The model under review builds one solid part; all positions refer to its coordinate system, in mm. A direction names the side the tool comes from. Give positions to 0.01 mm unless a question says otherwise; leave off trailing zeros. Loops run counter-clockwise (first coordinate to the right, second up) from the corner with the lowest first, then second, coordinate; pieces in that order, holes last. Notation, with made-up numbers: (71, 38) - (96, 38) arc R26 ccw to (96, 75) - close; hole circle Ø6 at (37.25, -18). An arc over 180 degrees is marked (long way). Return JSON: item names as keys, results as strings. Group by question number.
from build123d import *

# Parameters (mm, degrees)
BOX001_W        = 65
BOX001_H        = 34
BOX001_DEPTH    = 5
BOX_W           = 5
BOX_H           = 34
BOX_DEPTH       = 46
SKETCH_R        = 2.05
POCKET_DEPTH    = 5
SKETCH001_R     = 5
SKETCH001_R_2   = 1.7
POCKET001_DEPTH = 5
SKETCH002_R     = 4.5
POCKET002_DEPTH = 5
BOX002_W        = 44
BOX002_H        = 17
BOX002_DEPTH    = 78
SKETCH003_R     = 4
SKETCH003_R_2   = 1.5
POCKET003_DEPTH = 17.001
SKETCH004_W     = 44
SKETCH004_H     = 43
POCKET004_DEPTH = 1
SKETCH005_W     = 3
SKETCH005_H     = 13
PAD_DEPTH       = 17


with BuildPart() as cubo001:
    # Box001 → Box001 (new body)
    with BuildSketch(Plane(origin=(-30, -2, 46), x_dir=(1, 0, 0), z_dir=(0, 0, 1))):
        with Locations((32.5, 17)):
            Rectangle(BOX001_W, BOX001_H)
    extrude(amount=BOX001_DEPTH)


with BuildPart() as pocket002:
    # Box → Box (new body)
    with BuildSketch(Plane(origin=(0, -2, 0), x_dir=(1, 0, 0), z_dir=(0, 0, 1))):
        with Locations((2.5, 17)):
            Rectangle(BOX_W, BOX_H)
    extrude(amount=BOX_DEPTH)

    # Fusion: union Cubo001
    add(cubo001.part)

    # Sketch → Pocket (cut)
    with BuildSketch(Plane.XY.offset(51)):
        with Locations((-36.05, -7.05)):
            Circle(SKETCH_R)
        with Locations((28.95, 3.05)):
            Circle(SKETCH_R)
        with Locations((-55.15, -7.05)):
            Circle(SKETCH_R)
        with Locations((9.85, 3.05)):
            Circle(SKETCH_R)
        with Locations((-4.85, 3.05)):
            Circle(SKETCH_R)
        with Locations((-23.95, 3.05)):
            Circle(SKETCH_R)
        with Locations((-23.95, 26.95)):
            Circle(SKETCH_R)
        with Locations((-4.85, 26.95)):
            Circle(SKETCH_R)
        with Locations((9.85, 26.95)):
            Circle(SKETCH_R)
        with Locations((28.95, 26.95)):
            Circle(SKETCH_R)
    extrude(amount=-POCKET_DEPTH, mode=Mode.SUBTRACT)

    # Sketch001 → Pocket001 (cut)
    with BuildSketch(Plane.YZ.offset(5)):
        with Locations((15, 11)):
            Circle(SKETCH001_R)
        with Locations((15, 19.2)):
            Circle(SKETCH001_R_2)
        with Locations((23.2, 11)):
            Circle(SKETCH001_R_2)
        with Locations((15, 2.8)):
            Circle(SKETCH001_R_2)
        with Locations((6.8, 11)):
            Circle(SKETCH001_R_2)
    extrude(amount=-POCKET001_DEPTH, mode=Mode.SUBTRACT)

    # Sketch002 → Pocket002 (cut)
    with BuildSketch(Plane.YZ.offset(5)):
        with Locations((15, 34.8)):
            Circle(SKETCH002_R)
    extrude(amount=-POCKET002_DEPTH, mode=Mode.SUBTRACT)


with BuildPart() as fusion001002:
    # Box002 → Box002 (new body)
    with BuildSketch(Plane(origin=(-19.5, 15, 51), x_dir=(1, 0, 0), z_dir=(0, 0, 1))):
        with Locations((22, 8.5)):
            Rectangle(BOX002_W, BOX002_H)
    extrude(amount=BOX002_DEPTH)

    # Sketch003 → Pocket003 (cut, through all)
    with BuildSketch(Plane(origin=(-19.5, 15, 51), x_dir=(1, 0, 0), z_dir=(0, -1, 0))):
        with Locations((22, 6)):
            Circle(SKETCH003_R)
        with Locations((22, 63)):
            Circle(SKETCH003_R)
        with Locations((5.485017, 17)):
            Circle(SKETCH003_R_2)
        with Locations((38.514983, 17)):
            Circle(SKETCH003_R_2)
        with Locations((5.485017, 52)):
            Circle(SKETCH003_R_2)
        with Locations((38.514983, 52)):
            Circle(SKETCH003_R_2)
    extrude(amount=-POCKET003_DEPTH, mode=Mode.SUBTRACT)

    # Sketch004 → Pocket004 (cut)
    with BuildSketch(Plane(origin=(-19.5, 15, 51), x_dir=(1, 0, 0), z_dir=(0, -1, 0))):
        with Locations((22, 34.5)):
            Rectangle(SKETCH004_W, SKETCH004_H)
    extrude(amount=-POCKET004_DEPTH, mode=Mode.SUBTRACT)

    # Sketch005 → Pad (new body)
    with BuildSketch(Plane(origin=(-19.5, 15, 51), x_dir=(1, 0, 0), z_dir=(0, -1, 0))):
        with Locations((38.5, 6.5)):
            Rectangle(SKETCH005_W, SKETCH005_H)
        with Locations((5.5, 6.5)):
            Rectangle(SKETCH005_W, SKETCH005_H)
    extrude(amount=PAD_DEPTH)

    # Fusion001002: union Pocket002
    add(pocket002.part)


solid = fusion001002.part
Item 1: Mouldability with a two-part tool opening along X and no side actions: class faces 1 (the face through (2.535, 6.579, 12.686)), 2 (the face through (8.339, 4.435, 48.535)), 3 (the face through (5, 15, 23)) as +X half, -X half, draft (parallel to the pull), parting line (faces both ways), or undercut.
Item 2: Take a section at B-B (z = 103). State the section outline as (x, y) points, then the cut area to 3 significant figures.
Item 3: Take a section at C-C (z = 19.2). State the section outline as (x, y) points, then the cut area to 3 significant figures.
Item 4: For L1, parallel to Z at x = 2.5, y = 28; L2, parallel to X at y = 26.75, z = 68; L3, parallel to Y at x = 28, z = 47, list the stretches that pass through material, from the lowest coordinate up. Write a range as from..to.
Item 5: Tool access review of faces 4 (the face through (10, 27, 51)), 5 (the face through (-19.5, 23, 89)), 6 (the face through (2, 16, 86)), 7 (the face through (2, 15, 120)): name each direction out of +Z, -Z, +X, -X, +Y, -Y from which nothing blocks a thin tool from reaching the whole face with its end or side.
Item 6: Take a section at D-D (x = 28.95). State the section outline as (y, z) points, then the cut area to 3 significant figures.
Item 7: Take a section at A-A (y = 23.2). State the section outline as (x, z) points, then the cut area to 3 significant figures.
Item 8: For P1, Ø6, axis at x = -19, z = 115, coming from the -Y side; P2, Ø5.5, axis at x = -4.85, y = 3.05, coming from the -Z side; P3, Ø3.5, axis at x = 19.01, z = 68, coming from the -Y side, all flat-tipped, find the tip position at first contact; note any pin that passes through.
Check sheet entries:
{
 "1": {"face 1": "draft", "face 2": "undercut", "face 3": "+X half"},
 "2": {"outline": "(-19.5, 16) - (-15.51, 16) - (-15.51, 32) - (-19.5, 32) - close; (-12.51, 16) - (17.51, 16) - (17.51, 32) - (-12.51, 32) - close; (20.51, 16) - (24.5, 16) - (24.5, 32) - (20.51, 32) - close", "area": "608 mm^2"},
 "3": {"outline": "(0, -2) - (5, -2) - (5, 13.3) - (0, 13.3) - close; (0, 16.7) - (5, 16.7) - (5, 32) - (0, 32) - close", "area": "153 mm^2"},
 "4": {"L1": "z = 0..53, 61..110, 118..129", "L2": "x = -19.5..-15.51, -12.51..17.51, 20.51..24.5", "L3": "y = -2..1.23, 4.87..25.13, 28.77..32"},
 "5": {"face 4": "-Z", "face 5": "+Z, -X, +Y, -Y", "face 6": "+X, -X, -Y", "face 7": "+Z, +X, -X, -Y"},
 "6": {"outline": "(-2, 46) - (1, 46) - (1, 51) - (-2, 51) - close; (5.1, 46) - (24.9, 46) - (24.9, 51) - (5.1, 51) - close; (29, 46) - (32, 46) - (32, 51) - (29, 51) - close", "area": "129 mm^2"},
 "7": {"outline": "(-30, 46) - (0, 46) - (0, 12.7) - (5, 12.7) - (5, 46) - (35, 46) - (35, 51) - (24.5, 51) - (24.5, 129) - (-19.5, 129) - (-19.5, 51) - (-30, 51) - close; (0, 0) - (5, 0) - (5, 9.3) - (0, 9.3) - close; hole circle Ø3 at (-14.01, 68); hole circle Ø3 at (-14.01, 103); hole circle Ø8 at (2.5, 57); hole circle Ø8 at (2.5, 114); hole circle Ø3 at (19.01, 68); hole circle Ø3 at (19.01, 103)", "area": "3,840 mm^2"},
 "8": {"P1": "stops at y = 15", "P2": "stops at z = 46", "P3": "stops at y = 16"}
}
